```python
from build123d import *

# Parameters (mm, degrees)
SKETCH1_W           = 109
SKETCH1_H           = 50
SKETCH1_R           = 1.75
BOSS_EXTRUDE1_DEPTH = 2
FILLET1_R           = 2


with BuildPart() as part:
    # Sketch1 → Boss-Extrude1 (new body)
    with BuildSketch(Plane.XY):
        Rectangle(SKETCH1_W, SKETCH1_H)
        with Locations((-4.5, 20.5)):
            Circle(SKETCH1_R, mode=Mode.SUBTRACT)
        with Locations((-4.5, -20.5)):
            Circle(SKETCH1_R, mode=Mode.SUBTRACT)
        with Locations((-50, 20.5)):
            Circle(SKETCH1_R, mode=Mode.SUBTRACT)
        with Locations((-50, -20.5)):
            Circle(SKETCH1_R, mode=Mode.SUBTRACT)
        with Locations((50, -20.5)):
            Circle(SKETCH1_R, mode=Mode.SUBTRACT)
        with Locations((4.5, -20.5)):
            Circle(SKETCH1_R, mode=Mode.SUBTRACT)
        with Locations((4.5, 20.5)):
            Circle(SKETCH1_R, mode=Mode.SUBTRACT)
        with Locations((50, 20.5)):
            Circle(SKETCH1_R, mode=Mode.SUBTRACT)
        Polygon((-51.673539091, 18.642779789), (-30.984600544, 0), (-51.673539091, -18.642779789), align=None, mode=Mode.SUBTRACT)
        Polygon((-48.326460909, 22.357220211), (-27.25, 3.365244447), (-6.173539091, 22.357220211), align=None, mode=Mode.SUBTRACT)
        Polygon((-2.826460909, 18.642779789), (-2.826460909, -18.642779789), (-23.515399456, 0), align=None, mode=Mode.SUBTRACT)
        Polygon((-6.173539091, -22.357220211), (-48.326460909, -22.357220211), (-27.25, -3.365244447), align=None, mode=Mode.SUBTRACT)
        Polygon((6.173539091, -22.357220211), (48.326460909, -22.357220211), (27.25, -3.365244447), align=None, mode=Mode.SUBTRACT)
        Polygon((51.673539091, 18.642779789), (51.673539091, -18.642779789), (30.984600544, 0), align=None, mode=Mode.SUBTRACT)
        Polygon((48.326460909, 22.357220211), (6.173539091, 22.357220211), (27.25, 3.365244447), align=None, mode=Mode.SUBTRACT)
        Polygon((23.515399456, 0), (2.826460909, -18.642779789), (2.826460909, 18.642779789), align=None, mode=Mode.SUBTRACT)
    extrude(amount=BOSS_EXTRUDE1_DEPTH)

    # Fillet1
    fillet1_edges = [part.edges().sort_by_distance(p)[0] for p in [
        (27.25, 3.365244447, 1),
        (48.326460909, 22.357220211, 1),
        (6.173539091, 22.357220211, 1),
        (23.515399456, 0, 1),
        (2.826460909, 18.642779789, 1),
        (2.826460909, -18.642779789, 1),
        (-27.25, 3.365244447, 1),
        (-6.173539091, 22.357220211, 1),
        (-48.326460909, 22.357220211, 1),
        (-51.673539091, 18.642779789, 1),
        (-51.673539091, -18.642779789, 1),
        (-30.984600544, 0, 1),
        (-6.173539091, -22.357220211, 1),
        (-27.25, -3.365244447, 1),
        (-48.326460909, -22.357220211, 1),
        (-2.826460909, 18.642779789, 1),
        (-23.515399456, 0, 1),
        (-2.826460909, -18.642779789, 1),
        (54.5, -25, 1),
        (-54.5, -25, 1),
        (-54.5, 25, 1),
        (54.5, 25, 1),
        (27.25, -3.365244447, 1),
        (6.173539091, -22.357220211, 1),
        (48.326460909, -22.357220211, 1),
        (51.673539091, 18.642779789, 1),
        (30.984600544, 0, 1),
        (51.673539091, -18.642779789, 1),
    ]]
    fillet(fillet1_edges, radius=FILLET1_R)


solid = part.part
```
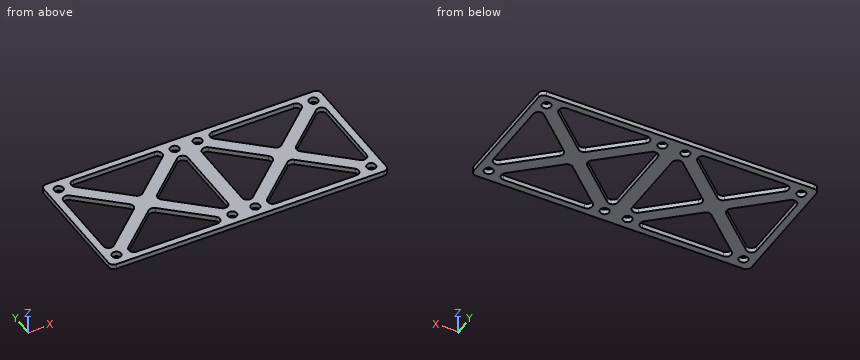
CAD build for the part. Positions are in the model's coordinates, mm. Coordinates: 2 decimals unless noted, no trailing zeros. Loops run counter-clockwise (first coordinate to the right, second up) from the corner with the lowest first, then second, coordinate; pieces in that order, holes last. Notation, with made-up numbers: (14, 36.25) - (23, 36.25) arc R14 ccw to (23, 56.25) - close; hole circle Ø2 at (38, 2.25). An arc over 180 degrees is marked (long way). Return JSON: item names as keys, results as strings.
1. Drop a flat-ended pin along its axis: pin 1 (3 mm diameter, centred on x = -50, y = -20.5, fed in from +Z). Give the stop position or say it passes through.
Result:
{"pin 1": "passes through"}
2. Band-saw the part on D-D (x = -4.5). Give the cut face in (y, z), and give its area (3 significant figures).
Result:
{"outline": "(-25, 0) - (-22.25, 0) - (-22.25, 2) - (-25, 2) - close; (-18.75, 0) - (-16.12, 0) - (-16.12, 2) - (-18.75, 2) - close; (16.12, 0) - (18.75, 0) - (18.75, 2) - (16.12, 2) - close; (22.25, 0) - (25, 0) - (25, 2) - (22.25, 2) - close", "area": "21.5 mm2"}
3. Probe L1, parallel to Y at x = 27, z = 1.75; L2, parallel to Y at x = 4.5, z = 0.65; L3, parallel to Y at x = 21, z = 1.15. List the from-to ranges inside material, lowest first. Write a range as from..to.
Result:
{"L1": "y = -25..-22.36, -4.07..4.07, 22.36..25", "L2": "y = -25..-22.25, -18.75..-16.12, 16.12..18.75, 22.25..25", "L3": "y = -25..-22.36, -9..-2.27, 2.27..9, 22.36..25"}
4. Band-saw the part on B-B (x = 17). Give the cut face in (y, z), and give its area (3 significant figures).
Result:
{"outline": "(-25, 0) - (-22.36, 0) - (-22.36, 2) - (-25, 2) - close; (-12.6, 0) - (-5.87, 0) - (-5.87, 2) - (-12.6, 2) - close; (5.87, 0) - (12.6, 0) - (12.6, 2) - (5.87, 2) - close; (22.36, 0) - (25, 0) - (25, 2) - (22.36, 2) - close", "area": "37.5 mm2"}
5. Band-saw the part on C-C (z = 1.7). State how many separate pieces and enclosed holes the cut face has, and give its area (3 significant figures).
Result:
{"separate pieces": "1", "enclosed holes": "16", "area": "2,310 mm2"}
6. Band-saw the part on A-A (y = -20.5). Give the cut face in (x, z), and give its area (3 significant figures).
Result:
{"outline": "(-54.5, 0) - (-51.75, 0) - (-51.75, 2) - (-54.5, 2) - close; (-48.25, 0) - (-45.11, 0) - (-45.11, 2) - (-48.25, 2) - close; (-9.39, 0) - (-6.25, 0) - (-6.25, 2) - (-9.39, 2) - close; (-2.75, 0) - (2.75, 0) - (2.75, 2) - (-2.75, 2) - close; (6.25, 0) - (9.39, 0) - (9.39, 2) - (6.25, 2) - close; (45.11, 0) - (48.25, 0) - (48.25, 2) - (45.11, 2) - close; (51.75, 0) - (54.5, 0) - (54.5, 2) - (51.75, 2) - close", "area": "47.1 mm2"}
